```python
from build123d import *

# Parameters (mm, degrees)
CORTAR_EXTRUIR1_DEPTH = 2.5
CHAFL_N1_SIZE         = 1


with BuildPart() as part:
    # Croquis1 → Revolución1 (revolve)
    with BuildSketch(Plane.XY):
        Polygon((-23.114362081, 0), (23.114362081, 0), (23.114362081, -3.175), (88.311435021, -3.175), (88.311435021, -12.7), (-59.557840342, -12.7), (-59.557840342, -3.175), (-23.114362081, -3.175), align=None)
    revolve(axis=Axis((88.311435021, -12.7, 0), (-1, 0, 0)))

    # Croquis2 → Cortar-Extruir1 (cut)
    with BuildSketch(Plane(origin=(0, -3.175, 0), x_dir=(1, 0, 0), z_dir=(0, 1, 0))):
        with BuildLine():
            Line((48.311435021, 2.38125), (88.311435021, 2.38125))
            ThreePointArc((88.311435021, 2.38125), (90.692685021, 0), (88.311435021, -2.38125))
            Line((88.311435021, -2.38125), (48.311435021, -2.38125))
            ThreePointArc((48.311435021, -2.38125), (45.930185021, 0), (48.311435021, 2.38125))
        make_face()
        with BuildLine():
            Line((-59.557840342, 2.38125), (-29.557840342, 2.38125))
            ThreePointArc((-29.557840342, 2.38125), (-27.176590342, 0), (-29.557840342, -2.38125))
            Line((-29.557840342, -2.38125), (-59.557840342, -2.38125))
            ThreePointArc((-59.557840342, -2.38125), (-61.939090342, 0), (-59.557840342, 2.38125))
        make_face()
    extrude(amount=-CORTAR_EXTRUIR1_DEPTH, mode=Mode.SUBTRACT)

    # Chaflán1
    chafl_n1_edges = [part.edges().sort_by_distance(p)[0] for p in [
        (88.311435021, -22.225, 0),
        (-59.557840342, -22.225, 0),
        (23.114362081, -25.4, 0),
        (-23.114362081, -25.4, 0),
    ]]
    chamfer(chafl_n1_edges, length=CHAFL_N1_SIZE)


solid = part.part
```
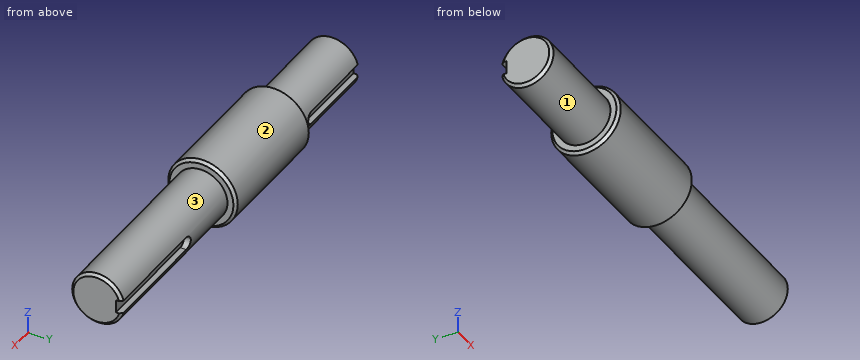
Model file for the job. Use its own axes, mm. Face numbers are marked on the shaded views. A direction names the side the tool comes from. Round coordinates to 2 decimals unless told otherwise and drop trailing zeros. Write each loop counter-clockwise with the first axis right and the second up, starting at its lowest first coordinate (ties: lowest second). Pieces come first, ordered by that corner, then holes. Notation, with made-up numbers: (-2.5, 31.25) - (31.5, 31.25) arc R35 cw to (31.5, 63.25) - close; hole circle Ø1 at (87, 9.25). An arc over 180 degrees is marked (long way). Use CSV: the item, a comma, the result in double quotes. Start each with the question number.
Item 1: Band-saw the part on D-D (x = 19). Write the cut outline in (y, z).
Item 2: Pin check, flat tips, straight feed: P1, Ø1.5, axis at x = 33.5, z = 3, coming from the +Y side; P2, Ø10, axis at x = -43.5, z = 7.5, coming from the -Y side; P3, Ø2.5, axis at x = 63, y = -5, coming from the +Z side. Stop position of each tip, or through.
Item 3: Band-saw the part on C-C (x = 36). Write the cut outline in (y, z) (3 decimals), and give its area (3 significant figures).
Item 4: Drill centre lines: L1, parallel to Z at x = 79.5, y = -12.25; L2, parallel to Z at x = 39.5, y = -10.5; L3, parallel to X at y = -18, z = 8. Where is each one in solid material? Low to high. Write a range as [from, to].
Item 5: Band-saw the part on A-A (y = -12.7). Write the cut outline in (x, z) (3 decimals), and give its area (3 significant figures).
Item 6: Tool access for the marked faces 1, 2 and 3: list every direction of +Z, -Z, +X, -X, +Y, -Y with a clear straight run to the whole face (end or side of a thin tool).
Item 7: Band-saw the part on B-B (z = 0). Write the cut outline in (x, y) (3 decimals), and give its area (3 significant figures).
Checked values:
1,outline,"circle Ø25.4 at (-12.7, 0)"
2,P1,"stops at y = -3.44"
2,P2,"stops at y = -21.89"
2,P3,"stops at z = 7.01"
3,outline,"circle Ø19.05 at (-12.7, 0)"
3,area,"285 mm²"
4,L1,"z = [-9.51, 9.51]"
4,L2,"z = [-9.27, 9.27]"
4,L3,"x = [-23.11, 23.11]"
5,outline,"(-59.558, -8.525) - (-58.558, -9.525) - (-23.114, -9.525) - (-23.114, -11.7) - (-22.114, -12.7) - (22.114, -12.7) - (23.114, -11.7) - (23.114, -9.525) - (87.311, -9.525) - (88.311, -8.525) - (88.311, 8.525) - (87.311, 9.525) - (23.114, 9.525) - (23.114, 11.7) - (22.114, 12.7) - (-22.114, 12.7) - (-23.114, 11.7) - (-23.114, 9.525) - (-58.558, 9.525) - (-59.558, 8.525) - close"
5,area,"3,110 mm²"
6,face 1,"-X"
6,face 2,"+X, -X"
6,face 3,"+X"
7,outline,"(-59.558, -21.225) - (-58.558, -22.225) - (-23.114, -22.225) - (-23.114, -24.4) - (-22.114, -25.4) - (22.114, -25.4) - (23.114, -24.4) - (23.114, -22.225) - (87.311, -22.225) - (88.311, -21.225) - (88.311, -5.675) - (45.93, -5.675) - (45.93, -3.175) - (23.114, -3.175) - (23.114, -1) - (22.114, 0) - (-22.114, 0) - (-23.114, -1) - (-23.114, -3.175) - (-27.177, -3.175) - (-27.177, -5.675) - (-59.558, -5.675) - close"
7,area,"2,920 mm²"
